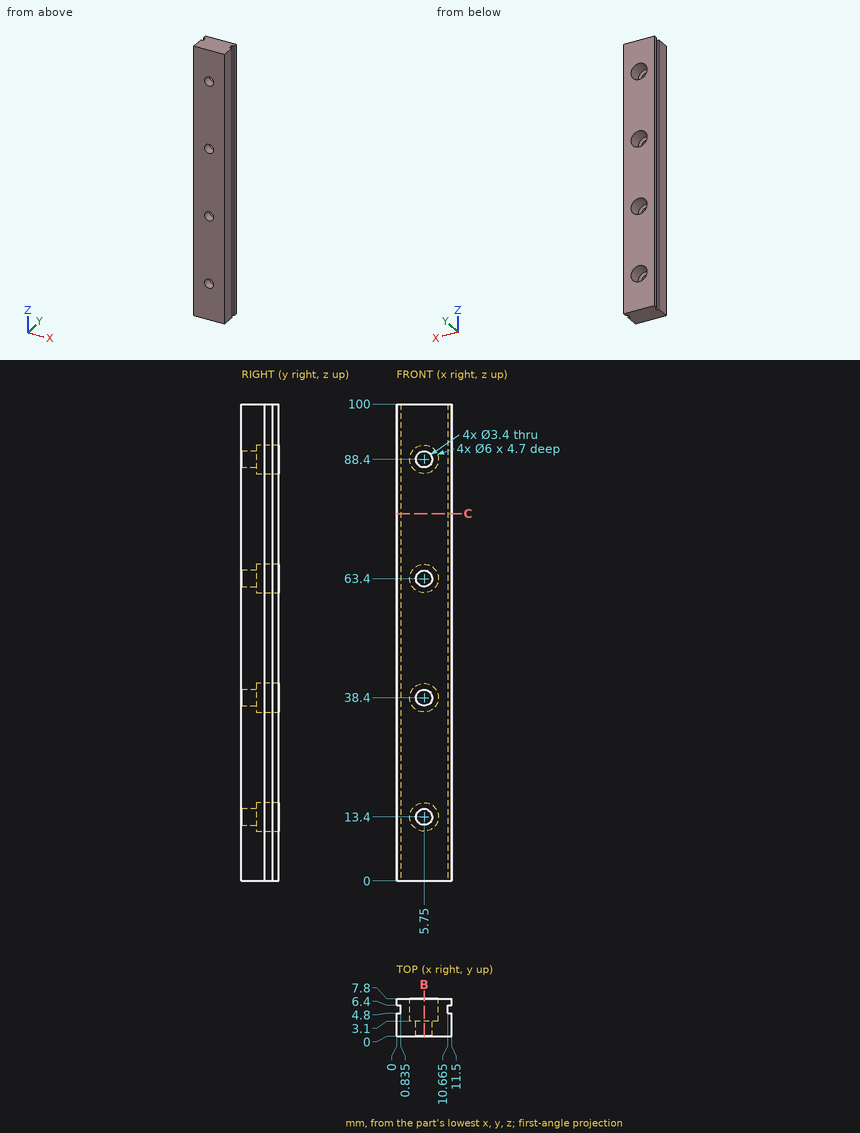
Verification items for this drawing (mm, ordinates from the low corner). Round coordinates to 2 decimals unless told otherwise and drop trailing zeros. Loops run counter-clockwise (first coordinate to the right, second up) from the corner with the lowest first, then second, coordinate; pieces in that order, holes last. Notation, with made-up numbers: (85.5, 56) -> (134.5, 56) arc R12 cw to (134.5, 68) -> close; hole circle Ø9 at (32.25, 31). An arc over 180 degrees is marked (long way). Write item = value, one per line. Start each with the question number.
1) Gauge pin test, flat ends, axial feed: pin 1 Ø1.8 at (x, z) = (7, 63) entering from +Y; pin 2 Ø2 at (x, z) = (5.75, 38.4) entering from -Y. Record the tip position at first contact, or that the pin passes through.
2) Thickness scan on probe 1 along Z at (x, y) = (5.5, 1); probe 2 along X at (y, z) = (1, 13.4); probe 3 along Z at (x, y) = (6.5, 7) (1 decimal). Record the ranges inside material, lowest first.
3) Sectioned sample at B-B, the plane x = 5.75. State how many separate pieces and enclosed holes the cut face has, plus the area to 3 significant figures.
4) Sectioned sample at C-C, the plane z = 77. Record the cut outline in (x, y) (1 decimal).
Results are:
q1.pin_1 = 3.1
q1.pin_2 = through
q2.probe_1 = 0 to 11.72, 15.08 to 36.72, 40.08 to 61.72, 65.08 to 86.72, 90.08 to 100
q2.probe_2 = 0 to 4.05, 7.45 to 11.5
q2.probe_3 = 0 to 10.5, 16.3 to 35.5, 41.3 to 60.5, 66.3 to 85.5, 91.3 to 100
q3.separate_pieces = 5
q3.enclosed_holes = 0
q3.area = 625 mm^2
q4.outline = (0, 0) -> (11.5, 0) -> (11.5, 4.8) -> (10.7, 4.8) -> (10.7, 6.4) -> (11.5, 6.4) -> (11.5, 7.8) -> (0, 7.8) -> (0, 6.4) -> (0.8, 6.4) -> (0.8, 4.8) -> (0, 4.8) -> close
